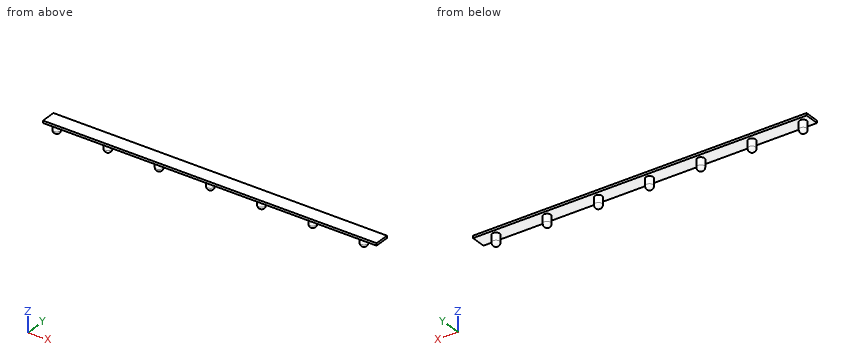
```python
from build123d import *

# Parameters (mm, degrees)
F0_W     = 228
F0_H     = 10
F1_DEPTH = 1.6
F2_R     = 2.5
F3_DEPTH = 7.5
F4_R     = 2.5


with BuildPart() as f1:
    # F0 (on Top) → F1 (new body)
    with BuildSketch(Plane.XY):
        Rectangle(F0_W, F0_H)
    extrude(amount=F1_DEPTH)

    # F2 (on face) → F3 (join)
    with BuildSketch(Plane(origin=(0, 0, 0), x_dir=(1, 0, 0), z_dir=(0, 0, -1))):
        with Locations((-108.5, -0.5)):
            Circle(F2_R)
        with Locations((-73.5, -0.5)):
            Circle(F2_R)
        with Locations((-38.5, -0.5)):
            Circle(F2_R)
        with Locations((-3.5, -0.5)):
            Circle(F2_R)
        with Locations((31.5, -0.5)):
            Circle(F2_R)
        with Locations((66.5, -0.5)):
            Circle(F2_R)
        with Locations((101.5, -0.5)):
            Circle(F2_R)
    extrude(amount=F3_DEPTH)

    # F4
    f4_edges = [f1.edges().sort_by_distance(p)[0] for p in [
        (-111, 0.5, -7.5),
        (-76, 0.5, -7.5),
        (-41, 0.5, -7.5),
        (-6, 0.5, -7.5),
        (29, 0.5, -7.5),
        (64, 0.5, -7.5),
        (99, 0.5, -7.5),
    ]]
    fillet(f4_edges, radius=F4_R)


solid = f1.part
```
Geometry check sheet. Reference: the model listing, model coordinates, mm. Round coordinates to 2 decimals unless told otherwise and drop trailing zeros. Order: outer loops, then holes, each group sorted by start corner. A loop starts at its lowest first (then second) coordinate and runs counter-clockwise, first axis right, second up. Notation, with made-up numbers: M 73,-39 L 97,-39 A25 ccw 97,-27 Z; hole C 26.25,-29.5 d6. An arc over 180 degrees is marked long. Answer as CSV lines item,"result".
1) Thickness scan on probe 1 along Z at (x, y) = (89, 3.75); probe 2 along Y at (x, z) = (31.5, -6.5); probe 3 along Y at (x, z) = (99.5, -1.75). Record the ranges inside material, lowest first. Write a range as [from, to].
Entries:
probe 1,"[0, 1.6]"
probe 2,"[-1.5, 2.5]"
probe 3,"[-1, 2]"
2) Sectioned sample at D-D on x = 94. Record the cut outline in (y, z).
Entries:
outline,"M -5,0 L 5,0 L 5,1.6 L -5,1.6 Z"
3) Sectioned sample at C-C on x = -73.5. Record the cut outline in (y, z), and give its area (3 significant figures).
Entries:
outline,"M -5,0 L -2,0 L -2,-5 A2.5 ccw 3,-5 L 3,0 L 5,0 L 5,1.6 L -5,1.6 Z"
area,"50.8 mm2"
4) Gauge pin test, flat ends, axial feed: pin 1 Ø3 at (x, y) = (57, 1) entering from -Z; pin 2 Ø5 at (x, z) = (3.5, -4) entering from -Y. Record the tip position at first contact, or that the pin passes through.
Entries:
pin 1,"z = 0"
pin 2,"through"
5) Sectioned sample at A-A on z = -2. Record the cut outline in (x, y), and give its area (3 significant figures).
Entries:
outline,"C -108.5,0.5 d5; C -73.5,0.5 d5; C -38.5,0.5 d5; C -3.5,0.5 d5; C 31.5,0.5 d5; C 66.5,0.5 d5; C 101.5,0.5 d5"
area,"137 mm2"
